Design review of the part shown in the three views and the two pictorial views. Dimensions are in mm from the part's minimum x, y and z. Coordinates: 2 decimals unless noted, no trailing zeros. Write each loop counter-clockwise with the first axis right and the second up, starting at its lowest first coordinate (ties: lowest second). Pieces come first, ordered by that corner, then holes. Notation, with made-up numbers: (-16.75, -11.75) -> (4.25, -11.75) arc R32 ccw to (4.25, 19.25) -> close; hole circle Ø9 at (64.5, -20). An arc over 180 degrees is marked (long way). Write item = value, one per line. Start each with the question number.
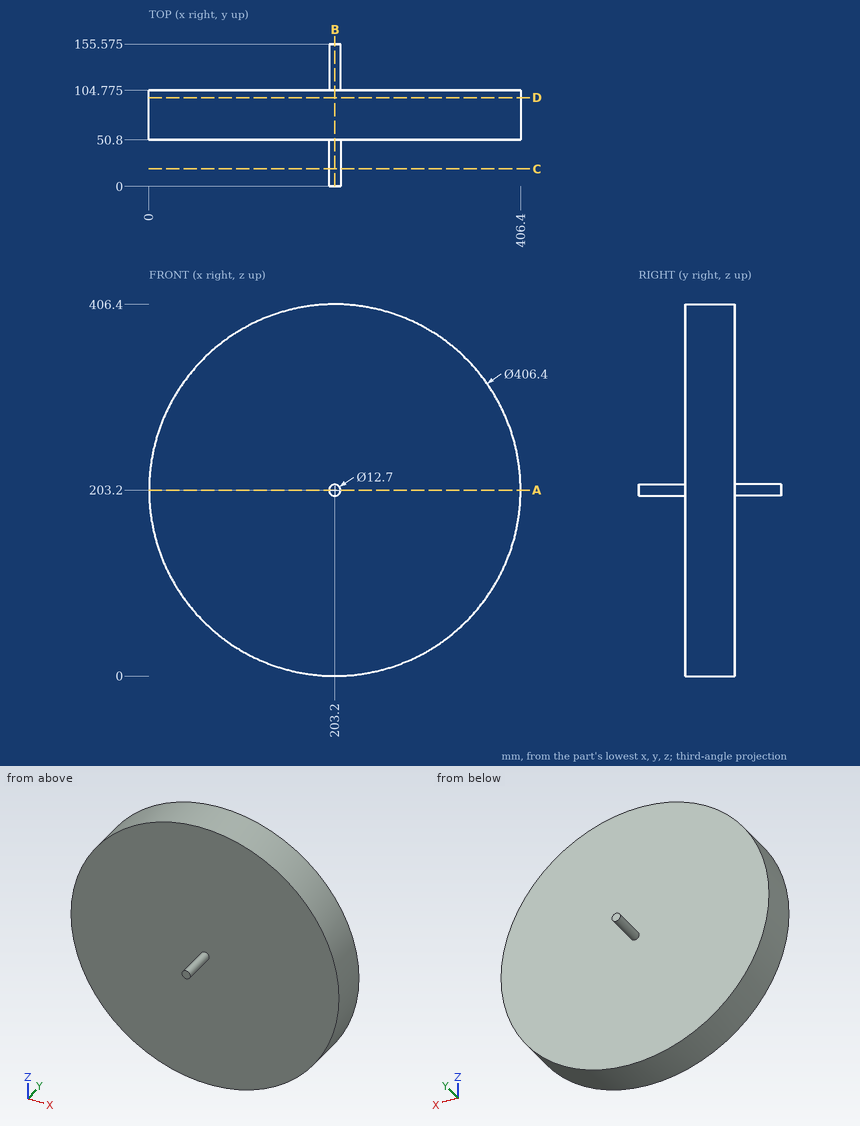
(1) Take a section at B-B, the plane x = 203.2. State the section outline as (y, z) points (3 decimals).
(2) Take a section at C-C, the plane y = 19. State the section outline as (x, z) points.
(3) For pin 1 Ø5 at (x, y) = (150, 69.5) entering from -Z; pin 2 Ø12 at (x, z) = (113, 328) entering from -Y; pin 3 Ø3 at (y, z) = (51, 345) entering from -X, all flat-tipped, find the tip position at first contact; note any pin that passes through.
(4) For line 1 (Y direction, x = 129, z = 277) (3 decimals); line 2 (Z direction, x = 218.5, y = 71); line 3 (X direction, y = 56.5, z = 248.5), list the stretches that pass through material, from the lowest coordinate up.
(5) Take a section at D-D, the plane y = 97. State the section outline as (x, z) points, then the cut area to 3 significant figures.
(6) Take a section at A-A, the plane z = 203.2. State the section outline as (x, y) points (3 decimals), then the cut area to 3 significant figures.
Report:
q1.outline = (0, 196.85) -> (50.8, 196.85) -> (50.8, 0) -> (104.775, 0) -> (104.775, 196.85) -> (155.575, 196.85) -> (155.575, 209.55) -> (104.775, 209.55) -> (104.775, 406.4) -> (50.8, 406.4) -> (50.8, 209.55) -> (0, 209.55) -> close
q2.outline = circle Ø12.7 at (203.2, 203.2)
q3.pin_1 = 6.43
q3.pin_2 = 50.8
q3.pin_3 = 56.21
q4.line_1 = 50.8 to 104.775
q4.line_2 = 0.58 to 405.82
q4.line_3 = 5.11 to 401.29
q5.outline = circle Ø406.4 at (203.2, 203.2)
q5.area = 130,000 mm2
q6.outline = (0, 50.8) -> (196.85, 50.8) -> (196.85, 0) -> (209.55, 0) -> (209.55, 50.8) -> (406.4, 50.8) -> (406.4, 104.775) -> (209.55, 104.775) -> (209.55, 155.575) -> (196.85, 155.575) -> (196.85, 104.775) -> (0, 104.775) -> close
q6.area = 23,200 mm2
